Could you check a few things on this model? Use its own coordinates, in mm. A direction names the side the tool comes from. Coordinates: 2 decimals unless noted, no trailing zeros. Write each loop counter-clockwise with the first axis right and the second up, starting at its lowest first coordinate (ties: lowest second). Pieces come first, ordered by that corner, then holes. Notation, with made-up numbers: (-21.5, 41) - (35.5, 41) arc R27 cw to (35.5, 62) - close; hole circle Ø6 at (33, -1). An arc over 180 degrees is marked (long way). Answer as a JSON object with one key per item and string values. Group by question number.
1) Please list where these lines run through material, in increasing order: line 1 along Z through (x, y) = (8, 2); line 2 along Z through (x, y) = (8, 0.95); line 3 along X through (y, z) = (2.2, -21).
2) On a 3-axis mill with a long thin cutter (end or side, diameter ignored), from which of +Z, -Z, +X, -X, +Y, -Y can I reach the whole of each face in a straight line? I mean faces 4 (the cylindrical face through (10.91, 0.28, -24.91)), 5 (the cylindrical face through (7.38, 2.19, -18.22)), 6 (the cylindrical face through (2.177, 0.285, -24.699)). Say none if no direction works.
3) If we section it at A-A (z = -21): Write out the boundary of the cut face in (x, y).
4) Will these pins go through, and if not, where does the flat tip stop? pin 1 Ø1.7 at (x, z) = (9, -9) entering from +Y; pin 2 Ø4.5 at (x, z) = (8.5, -20) entering from +Y.
5) If we section it at B-B (x = 8): Write out the boundary of the cut face in (y, z).
6) If we section it at C-C (y = 0.7): Write out the boundary of the cut face in (x, z), plus the area to 3 significant figures.
7) We'd pull the mould along Y, two halves only. Please class faces 1 (the flat face through (9.2, 1.35, -19.8)), 2 (the flat face through (7, 0, -13)), 3 (the flat face through (0, 1, -12)): released by +Y, released by -Y, zero draft, split by the parting line, or undercut.
8) If we section it at D-D (z = -9.25): Write out the boundary of the cut face in (x, y).
```python
from build123d import *

# Parameters (mm, degrees)
SKETCH1_W           = 14
SKETCH1_H           = 25
SKETCH1_R           = 1.5
BOSS_EXTRUDE1_DEPTH = 3
CHAMFER1_SIZE       = 0.5
FILLET1_R           = 1
SKETCH2_R           = 2.85
CUT_EXTRUDE1_DEPTH  = 1.65
BOSS_EXTRUDE2_START = -1
BOSS_EXTRUDE2_DEPTH = 1


with BuildPart() as part:
    # Sketch1 → Boss-Extrude1 (new body)
    with BuildSketch(Plane(origin=(0, 0, 0), x_dir=(1, 0, 0), z_dir=(0, 1, 0))):
        with Locations((7, 12.5)):
            Rectangle(SKETCH1_W, SKETCH1_H)
        with Locations((8, 21)):
            Circle(SKETCH1_R, mode=Mode.SUBTRACT)
        with Locations((8, 8.5895)):
            Circle(SKETCH1_R, mode=Mode.SUBTRACT)
    extrude(amount=BOSS_EXTRUDE1_DEPTH)

    # Chamfer1
    chamfer1_edges = [part.edges().sort_by_distance(p)[0] for p in [
        (14, 3, -12.5),
        (7, 3, -25),
        (0, 3, -12.5),
        (7, 3, 0),
    ]]
    chamfer(chamfer1_edges, length=CHAMFER1_SIZE)

    # Fillet1
    fillet1_edges = [part.edges().sort_by_distance(p)[0] for p in [
        (7, 0, -25),
        (7, 0, 0),
    ]]
    fillet(fillet1_edges, radius=FILLET1_R)

    # Sketch2 → Cut-Extrude1 (cut)
    with BuildSketch(Plane(origin=(0, 3, 0), x_dir=(1, 0, 0), z_dir=(0, 1, 0))):
        with Locations((8, 21)):
            Circle(SKETCH2_R)
        with Locations((8, 8.5895)):
            Circle(SKETCH2_R)
    extrude(amount=-CUT_EXTRUDE1_DEPTH, mode=Mode.SUBTRACT)

    # Sketch3 → Boss-Extrude2 (add)
    with BuildSketch(Plane.XZ.offset(BOSS_EXTRUDE2_START)):
        with BuildLine():
            ThreePointArc((4.5, -24), (4.792893219, -24.707106781), (5.5, -25))
            Line((5.5, -25), (10.5, -25))
            ThreePointArc((10.5, -25), (11.207106781, -24.707106781), (11.5, -24))
            Line((11.5, -24), (4.5, -24))
        make_face()
    extrude(amount=BOSS_EXTRUDE2_DEPTH)


solid = part.part
```
Here are the results:
{
 "1": {"line 1": "z = -25 to -23.85, -18.15 to -11.44, -5.74 to 0", "line 2": "z = -25 to -22.5, -19.5 to -10.09, -7.09 to 0", "line 3": "x = 0 to 5.15, 10.85 to 14"},
 "2": {"face 4": "-Z, +X, -Y", "face 5": "+Y", "face 6": "-Z, -X, -Y"},
 "3": {"outline": "(0, 0) - (6.5, 0) - (6.5, 1.35) - (5.15, 1.35) - (5.15, 3) - (0.5, 3) - (0, 2.5) - close; (9.5, 0) - (14, 0) - (14, 2.5) - (13.5, 3) - (10.85, 3) - (10.85, 1.35) - (9.5, 1.35) - close"},
 "4": {"pin 1": "stops at y = 1.35", "pin 2": "stops at y = 3"},
 "5": {"outline": "(0, -25) - (2.5, -25) - (3, -24.5) - (3, -23.85) - (1.35, -23.85) - (1.35, -22.5) - (0, -22.5) - close; (0, -19.5) - (1.35, -19.5) - (1.35, -18.15) - (3, -18.15) - (3, -11.44) - (1.35, -11.44) - (1.35, -10.09) - (0, -10.09) - close; (0, -7.09) - (1.35, -7.09) - (1.35, -5.74) - (3, -5.74) - (3, -0.5) - (2.5, 0) - (1, 0) arc R1 ccw to (0, -1) - close"},
 "6": {"outline": "(0, -24.95) - (5.2, -24.95) arc R1 ccw to (5.5, -25) - (10.5, -25) arc R1 ccw to (10.8, -24.95) - (14, -24.95) - (14, -0.05) - (0, -0.05) - close; hole circle Ø3 at (8, -21); hole circle Ø3 at (8, -8.59)", "area": "335 mm²"},
 "7": {"face 1": "released by +Y", "face 2": "released by -Y", "face 3": "zero draft"},
 "8": {"outline": "(0, 0) - (6.65, 0) - (6.65, 1.35) - (5.23, 1.35) - (5.23, 3) - (0.5, 3) - (0, 2.5) - close; (9.35, 0) - (14, 0) - (14, 2.5) - (13.5, 3) - (10.77, 3) - (10.77, 1.35) - (9.35, 1.35) - close"}
}
